CAD build for the part. Positions are in the model's coordinates, mm. A direction names the side the tool comes from. Give positions to 0.01 mm unless a question says otherwise; leave off trailing zeros. Write each loop counter-clockwise with the first axis right and the second up, starting at its lowest first coordinate (ties: lowest second). Pieces come first, ordered by that corner, then holes. Notation, with made-up numbers: (82.25, 79) - (130.25, 79) arc R30 cw to (130.25, 108) - close; hole circle Ø9 at (-16.5, 88). An arc over 180 degrees is marked (long way). Answer as a JSON object with one key per item and string values.
from build123d import *

# Parameters (mm, degrees)
F1_DEPTH = 2
F2_R     = 0.5
F3_DEPTH = 4
F4_SIZE  = 2
F5_R     = 0.5
F6_DEPTH = 8
F7_R     = 3


# Not quite as in the source:
# - a feature names something its author has since deleted; it is built from what else it names


with BuildPart() as f1:
    # F0 (on Top) → F1 (new body)
    with BuildSketch(Plane.XY):
        with BuildLine():
            Line((25.88854382, -10.5801345413), (40.4508497187, 0))
            Line((40.4508497187, 0), (25.88854382, 10.5801345413))
            ThreePointArc((25.88854382, 10.5801345413), (25.3831849379, 8.475163306), (23.5374028108, 7.3440665638))
            Line((23.5374028108, 7.3440665638), (25.6267504373, 5.8260666573))
            Line((25.6267504373, 5.8260666573), (33.6456432519, 0))
            Line((33.6456432519, 0), (10.7841511133, -16.6098462924))
            ThreePointArc((10.7841511133, -16.6098462924), (11.814451709, -18.3291218838), (12.94427191, -19.9846985779))
            Line((12.94427191, -19.9846985779), (22.6524758425, -12.9312755504))
            Line((22.6524758425, -12.9312755504), (25.88854382, -10.5801345413))
        make_face()
        with BuildLine():
            ThreePointArc((22.6524758425, -12.9312755504), (27.1085880869, -15.6619846459), (25.88854382, -10.5801345413))
            Line((25.88854382, -10.5801345413), (22.6524758425, -12.9312755504))
        make_face()
        with BuildLine():
            Line((25.6267504373, 5.8260666573), (23.5374028108, 7.3440665638))
            ThreePointArc((23.5374028108, 7.3440665638), (21.4324315756, 7.8494254458), (20.3013348333, 9.6952075729))
            Line((20.3013348333, 9.6952075729), (18.2119872068, 11.2132074794))
            ThreePointArc((18.2119872068, 11.2132074794), (20.1560130652, 6.0925860852), (25.6267504373, 5.8260666573))
        make_face()
        with BuildLine():
            Line((18.2119872068, 11.2132074794), (20.3013348333, 9.6952075729))
            ThreePointArc((20.3013348333, 9.6952075729), (20.8066937154, 11.8001788082), (22.6524758425, 12.9312755504))
            Line((22.6524758425, 12.9312755504), (12.94427191, 19.9846985779))
            ThreePointArc((12.94427191, 19.9846985779), (11.814451709, 18.3291218838), (10.7841511133, 16.6098462924))
            Line((10.7841511133, 16.6098462924), (18.2119872068, 11.2132074794))
        make_face()
    extrude(amount=F1_DEPTH)

    # F2
    f2_edges = [f1.edges().sort_by_distance(p)[0] for p in [
        (21.432432, 7.849425, 2),
    ]]
    fillet(f2_edges, radius=F2_R)



with BuildPart() as f1b:
    # F0 (on Top) → F1, piece 2 (new body)
    with BuildSketch(Plane.XY):
        with BuildLine():
            Line((0, -29.3892626146), (11.3262379212, -21.1602690825))
            ThreePointArc((11.3262379212, -21.1602690825), (10.1939633159, -19.506943), (9.1554367996, -17.7931765073))
            Line((9.1554367996, -17.7931765073), (0, -24.4449907046))
            Line((0, -24.4449907046), (-25.5664713255, -5.8698619956))
            ThreePointArc((-25.5664713255, -5.8698619956), (-26.4247321499, -7.6985729811), (-27.5065778087, -9.4045640367))
            Line((-27.5065778087, -9.4045640367), (-25.88854382, -10.5801345413))
            Line((-25.88854382, -10.5801345413), (-14.5623058987, -18.8091280734))
            Line((-14.5623058987, -18.8091280734), (0, -29.3892626146))
        make_face()
    extrude(amount=F1_DEPTH)


with BuildPart() as f1c:
    # F0 (on Top) → F1, piece 3 (new body)
    with BuildSketch(Plane.XY):
        with BuildLine():
            Line((9.1554367996, -17.7931765073), (10.7841511133, -16.6098462924))
            ThreePointArc((10.7841511133, -16.6098462924), (6.4508497187, 0), (10.7841511133, 16.6098462924))
            Line((10.7841511133, 16.6098462924), (9.1554367996, 17.7931765073))
            ThreePointArc((9.1554367996, 17.7931765073), (5.8461773909, 9.9255555553), (4.4821132939, 1.5))
            ThreePointArc((4.4821132939, 1.5), (4.4508497187, 0), (4.4821132939, -1.5))
            ThreePointArc((4.4821132939, -1.5), (5.8461773909, -9.9255555553), (9.1554367996, -17.7931765073))
        make_face()
    extrude(amount=F1_DEPTH)


with BuildPart() as f1d:
    # F0 (on Top) → F1, piece 4 (new body)
    with BuildSketch(Plane.XY):
        with BuildLine():
            ThreePointArc((-29.1246117975, -8.2289935321), (-28.0552509558, -6.5076210175), (-27.2456067433, -4.6498987043))
            Line((-27.2456067433, -4.6498987043), (-33.6456432519, 0))
            Line((-33.6456432519, 0), (-27.2456067433, 4.6498987043))
            ThreePointArc((-27.2456067433, 4.6498987043), (-28.0552509558, 6.5076210175), (-29.1246117975, 8.2289935321))
            Line((-29.1246117975, 8.2289935321), (-40.4508497187, 0))
            Line((-40.4508497187, 0), (-29.1246117975, -8.2289935321))
        make_face()
    extrude(amount=F1_DEPTH)


with BuildPart() as f1_1:
    add(f1.part)

    add(f1b.part)  # F3 merges F1b

    add(f1c.part)  # F3 merges F1c

    add(f1d.part)  # F3 merges F1d
    # F0 (on Top) → F3 (join)
    with BuildSketch(Plane.XY):
        with BuildLine():
            Line((-27.2456067433, -4.6498987043), (-25.5664713255, -5.8698619956))
            ThreePointArc((-25.5664713255, -5.8698619956), (-24.8897380342, -3.7218010616), (-24.5213173967, -1.5))
            ThreePointArc((-24.5213173967, -1.5), (-24.4508497187, 0), (-24.5213173967, 1.5))
            ThreePointArc((-24.5213173967, 1.5), (-24.7650379905, 3.1552037061), (-25.1802669457, 4.7759084761))
            ThreePointArc((-25.1802669457, 4.7759084761), (-25.3634508604, 5.3263867387), (-25.5664713255, 5.8698619956))
            Line((-25.5664713255, 5.8698619956), (-27.2456067433, 4.6498987043))
            ThreePointArc((-27.2456067433, 4.6498987043), (-26.4508497187, 0), (-27.2456067433, -4.6498987043))
        make_face()
        with BuildLine():
            Line((9.1554367996, -17.7931765073), (10.7841511133, -16.6098462924))
            ThreePointArc((10.7841511133, -16.6098462924), (6.4508497187, 0), (10.7841511133, 16.6098462924))
            Line((10.7841511133, 16.6098462924), (9.1554367996, 17.7931765073))
            ThreePointArc((9.1554367996, 17.7931765073), (5.8461773909, 9.9255555553), (4.4821132939, 1.5))
            ThreePointArc((4.4821132939, 1.5), (4.4508497187, 0), (4.4821132939, -1.5))
            ThreePointArc((4.4821132939, -1.5), (5.8461773909, -9.9255555553), (9.1554367996, -17.7931765073))
        make_face()
        with BuildLine():
            Line((11.3262379212, -21.1602690825), (12.94427191, -19.9846985779))
            ThreePointArc((12.94427191, -19.9846985779), (11.814451709, -18.3291218838), (10.7841511133, -16.6098462924))
            Line((10.7841511133, -16.6098462924), (9.1554367996, -17.7931765073))
            ThreePointArc((9.1554367996, -17.7931765073), (10.1939633159, -19.506943), (11.3262379212, -21.1602690825))
        make_face()
        with BuildLine():
            Line((9.1554367996, 17.7931765073), (10.7841511133, 16.6098462924))
            ThreePointArc((10.7841511133, 16.6098462924), (11.814451709, 18.3291218838), (12.94427191, 19.9846985779))
            Line((12.94427191, 19.9846985779), (11.3262379212, 21.1602690825))
            ThreePointArc((11.3262379212, 21.1602690825), (10.1939633159, 19.506943), (9.1554367996, 17.7931765073))
        make_face()
        with BuildLine():
            Line((-24.5213173967, -1.5), (-3.5491502813, -1.5))
            Line((-3.5491502813, -1.5), (-3.5491502813, 1.5))
            Line((-3.5491502813, 1.5), (-24.5213173967, 1.5))
            ThreePointArc((-24.5213173967, 1.5), (-24.4508497187, 0), (-24.5213173967, -1.5))
        make_face()
        with BuildLine():
            ThreePointArc((-27.5065778087, -9.4045640367), (-26.4247321499, -7.6985729811), (-25.5664713255, -5.8698619956))
            Line((-25.5664713255, -5.8698619956), (-27.2456067433, -4.6498987043))
            ThreePointArc((-27.2456067433, -4.6498987043), (-28.0552509558, -6.5076210175), (-29.1246117975, -8.2289935321))
            Line((-29.1246117975, -8.2289935321), (-27.5065778087, -9.4045640367))
        make_face()
        with BuildLine():
            ThreePointArc((-25.5664713255, 5.8698619956), (-26.4247321499, 7.6985729811), (-27.5065778087, 9.4045640367))
            Line((-27.5065778087, 9.4045640367), (-29.1246117975, 8.2289935321))
            ThreePointArc((-29.1246117975, 8.2289935321), (-28.0552509558, 6.5076210175), (-27.2456067433, 4.6498987043))
            Line((-27.2456067433, 4.6498987043), (-25.5664713255, 5.8698619956))
        make_face()
    extrude(amount=F3_DEPTH)

    # F4
    f4_edges = [f1_1.edges().sort_by_distance(p)[0] for p in [
        (12.135255, 20.572484, 4),
        (12.135255, -20.572484, 4),
    ]]
    chamfer(f4_edges, length=F4_SIZE)

    # F5
    f5_edges = [f1_1.edges().sort_by_distance(p)[0] for p in [
        (-26.45085, 0, 4),
        (11.00599, 18.920807, 4),
        (4.45085, 0, 4),
        (6.45085, 0, 4),
        (11.00599, -18.920807, 4),
    ]]
    fillet(f5_edges, radius=F5_R)

    # F0 (on Top) → F6 (join)
    with BuildSketch(Plane.XY):
        with BuildLine():
            Line((-3.5491502813, -1.5), (4.4821132939, -1.5))
            ThreePointArc((4.4821132939, -1.5), (4.4508497187, 0), (4.4821132939, 1.5))
            Line((4.4821132939, 1.5), (-3.5491502813, 1.5))
            Line((-3.5491502813, 1.5), (-3.5491502813, -1.5))
        make_face()
    extrude(amount=F6_DEPTH)

    # F7
    f7_edges = [f1_1.edges().sort_by_distance(p)[0] for p in [
        (4.45085, 0, 8),
        (-3.54915, 0, 8),
    ]]
    fillet(f7_edges, radius=F7_R)


solid = f1_1.part
Item 1: Cut at C-C (z = 6.5). Give the cut face in (x, y).
Entries:
{"outline": "(-3.15, -1.5) - (4.08, -1.5) arc R36.4 cw to (4.08, 1.5) - (-3.15, 1.5) - close"}
Item 2: Cut at B-B (x = -30). Give the cut face in (y, z), and give its area (3 significant figures).
Entries:
{"outline": "(-7.59, 0) - (-2.65, 0) - (-2.65, 2) - (-7.59, 2) - close; (2.65, 0) - (7.59, 0) - (7.59, 2) - (2.65, 2) - close", "area": "19.8 mm2"}
Item 3: Flat gauge pins, fed straight in: P1, Ø1.5, axis at x = 2, z = 6.5, coming from the +Y side; P2, Ø1.9, axis at x = 7, y = -1.5, coming from the +Z side; P3, Ø6, axis at x = -29.5, y = -13, coming from the -Z side; P4, Ø10.5, axis at x = -36, y = 0, coming from the +Z side. Where does each tip first touch, or does it go through?
Entries:
{"P1": "y = 1.5", "P2": "z = 4", "P3": "through", "P4": "z = 2"}
Item 4: Probe line 1 (X direction, y = -24, z = 1.5); line 2 (Z direction, x = 28.5, y = 5.5); line 3 (Y direction, x = -6, z = 1.75). List the from-to ranges inside material, lowest first. Write a range as from..to.
Entries:
{"line 1": "-7.42..-0.61, 0.61..7.42", "line 2": "0..2", "line 3": "-25.03..-20.09, -1.5..1.5"}
Item 5: Which spindle directions (+Z, -Z, +X, -X, +Y, -Y) get a long thin tool onto all of the face, cutting with end or side? Do faces 1 (the cylindrical face through (6.501, 11.975, 1.726)), 2 (the flat face through (6, -6, 0)), 3 (the cylindrical face through (-2.65, -0.02, 7.14)), 4 (the flat face through (33.068, -5.364, 0.986)), 5 (the flat face through (-30.49, 2.292, 0.986)). Say none if no direction does.
Entries:
{"face 1": "+Z, -Z, +Y", "face 2": "-Z, +X, -X, +Y, -Y", "face 3": "+Z, -X, +Y, -Y", "face 4": "+Z, -Z, +X", "face 5": "+Z, -Z"}
Item 6: Mould opens along Y. For faces 6 (the flat face through (-7, 1.5, 3)), 7 (the flat face through (-17, 0, 4)), 8 (the cylindrical face through (6.404, -11.696, 1.726)), 9 (the flat face through (22.37, -8.19, 0.99)) say: +Y half, -Y half, draft (parallel to the pull), parting line (faces both ways), or undercut.
Entries:
{"face 6": "+Y half", "face 7": "draft", "face 8": "undercut", "face 9": "undercut"}
Item 7: Cut at A-A (y = -22). Give the cut face in (x, z), and give its area (3 significant figures).
Entries:
{"outline": "(-10.17, 0) - (-3.37, 0) - (-3.37, 2) - (-10.17, 2) - close; (3.37, 0) - (10.17, 0) - (10.17, 2) - (3.37, 2) - close", "area": "27.2 mm2"}
